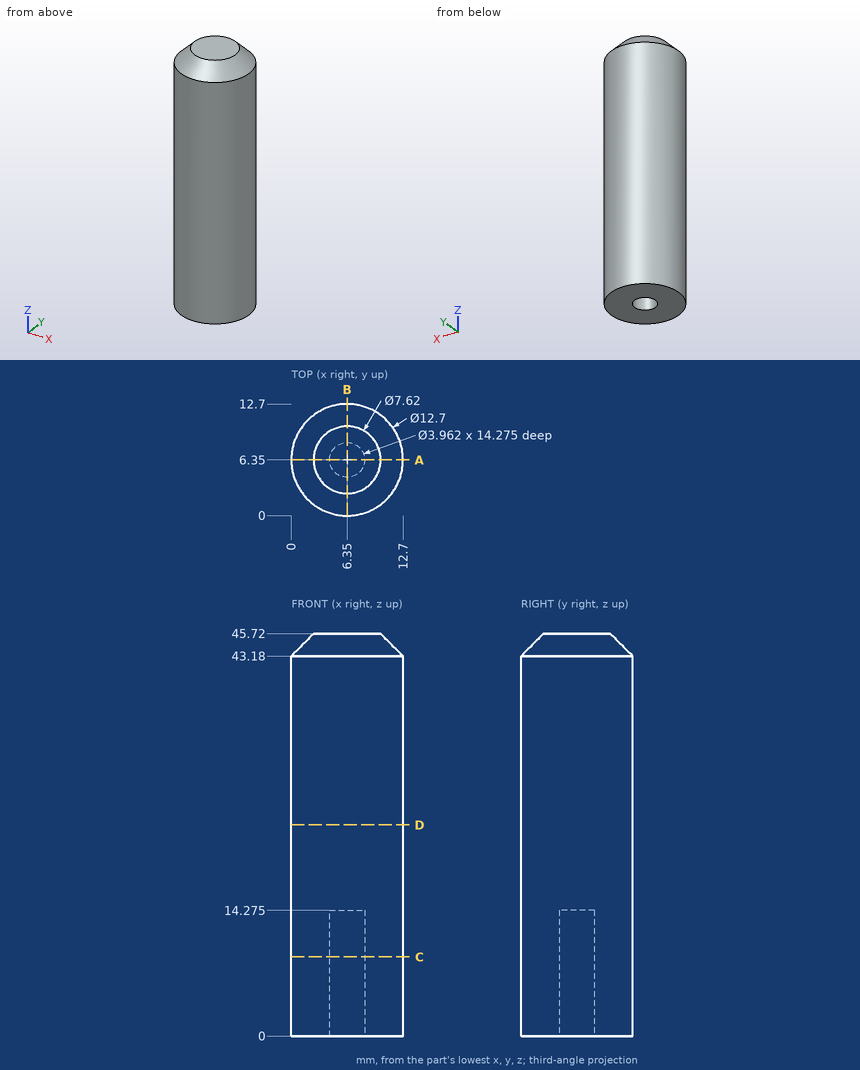
Verification items for this drawing (mm, ordinates from the low corner). Coordinates: 2 decimals unless noted, no trailing zeros. Write each loop counter-clockwise with the first axis right and the second up, starting at its lowest first coordinate (ties: lowest second). Pieces come first, ordered by that corner, then holes. Notation, with made-up numbers: M 62.25,22.5 L 70.25,22.5 A35 ccw 70.25,54.5 Z; hole C 54,-9.5 d3. An arc over 180 degrees is marked long. One line per item, written item: value. Start each with the question number.
(1) Sectioned sample at D-D, the plane z = 24. Enter the section's corners in (x, y), and give its area (3 significant figures).
(2) Scan lines: line 1 along Y through (x, z) = (6.35, 8.75); line 2 along X through (y, z) = (6.25, 37); line 3 along Z through (x, y) = (6, 5) (1 decimal). Record each from-to range of solid material in increasing order. Write a range as [from, to].
(3) Sectioned sample at A-A, the plane y = 6.35. Enter the section's corners in (x, z) (1 decimal).
(4) Sectioned sample at C-C, the plane z = 9. Enter the section's corners in (x, y), and give its area (3 significant figures).
(5) Depth check by flat-ended pin: pin 1 (2.5 mm diameter, centred on x = 6.35, y = 6.35, fed in from -Z) (1 decimal); pin 2 (3 mm diameter, centred on x = 4.5, z = 16.5, fed in from -Y); pin 3 (1.5 mm diameter, centred on x = 3.5, z = 24, fed in from -Y). Enter the tip coordinate at first touch or a pass-through.
Filled sheet:
1. outline: C 6.35,6.35 d12.7
1. area: 127 mm²
2. line 1: [0, 4.37], [8.33, 12.7]
2. line 2: [0, 12.7]
2. line 3: [14.3, 45.7]
3. outline: M 0,0 L 4.4,0 L 4.4,14.3 L 8.3,14.3 L 8.3,0 L 12.7,0 L 12.7,43.2 L 10.2,45.7 L 2.5,45.7 L 0,43.2 Z
4. outline: C 6.35,6.35 d12.7; hole C 6.35,6.35 d3.96
4. area: 114 mm²
5. pin 1: z = 14.3
5. pin 2: y = 0.01
5. pin 3: y = 0.36
